Work out the finished part from the listing and answer in its coordinate system (mm). Round coordinates to 2 decimals unless told otherwise and drop trailing zeros. Write each loop counter-clockwise with the first axis right and the second up, starting at its lowest first coordinate (ties: lowest second). Pieces come first, ordered by that corner, then holes. Notation, with made-up numbers: (73.25, 60) -> (116.25, 60) arc R33 ccw to (116.25, 96) -> close; hole circle Ø5 at (1, 35.25). An arc over 180 degrees is marked (long way). One line per question, with ' | ' between items. Start each with the question number.
Autodesk Inventor part; units mm, degrees
ref_plane "YZ Plane" through (0, 0, 0) normal (1, 0, 0) x (0, 1, 0)
ref_plane "XZ Plane" through (0, 0, 0) normal (0, 1, 0) x (-1, 0, 0)
ref_plane "XY Plane" through (0, 0, 0) normal (0, 0, 1) x (1, 0, 0)
sketch "Náčrt1" plane through (0, 0, 0) normal (0, 0, 1) x (1, 0, 0)
  line L0 (0, 75) -> (0, 5)
  line L1 (145, 80) -> (5, 80)
  line L2 (5, 0) -> (145, 0)
  line L3 (150, 5) -> (150, 75)
  line L4 (21.25, 29.75) -> (21.25, 66.25)
  line L5 (21.25, 66.25) -> (36.75, 66.25)
  line L6 (36.75, 66.25) -> (36.75, 29.75)
  line L7 (36.75, 29.75) -> (21.25, 29.75)
  line L8 (41.25, 29.75) -> (41.25, 66.25)
  line L9 (56.75, 29.75) -> (41.25, 29.75)
  line L10 (56.75, 66.25) -> (56.75, 29.75)
  line L11 (41.25, 66.25) -> (56.75, 66.25)
  line L12 (140, 36) -> (68.5, 36)
  line L13 (68.5, 36) -> (68.5, 60.5)
  line L14 (68.5, 60.5) -> (140, 60.5)
  line L15 (140, 60.5) -> (140, 36)
  line L16 (74.75, 19.75) -> (74.75, 24.25)
  line L17 (79.25, 24.25) -> (79.25, 19.75)
  line L18 (74.75, 24.25) -> (79.25, 24.25)
  line L19 (79.25, 19.75) -> (74.75, 19.75)
  line L20 (90.05, 19.75) -> (85.55, 19.75)
  line L21 (85.55, 19.75) -> (85.55, 24.25)
  line L22 (85.55, 24.25) -> (90.05, 24.25)
  line L23 (90.05, 24.25) -> (90.05, 19.75)
  line L24 (96.24, 19.75) -> (96.24, 24.25)
  line L25 (96.24, 24.25) -> (100.74, 24.25)
  line L26 (100.74, 19.75) -> (96.24, 19.75)
  line L27 (100.74, 24.25) -> (100.74, 19.75)
  line L28 (107.14, 19.75) -> (107.14, 24.25)
  line L29 (107.14, 24.25) -> (111.64, 24.25)
  line L30 (111.64, 19.75) -> (107.14, 19.75)
  line L31 (111.64, 24.25) -> (111.64, 19.75)
  line L32 (117.93, 19.75) -> (117.93, 24.25)
  line L33 (117.93, 24.25) -> (122.43, 24.25)
  line L34 (122.43, 19.75) -> (117.93, 19.75)
  line L35 (122.43, 24.25) -> (122.43, 19.75)
  line L36 (128.74, 19.75) -> (128.74, 24.25)
  line L37 (128.74, 24.25) -> (133.24, 24.25)
  line L38 (133.24, 19.75) -> (128.74, 19.75)
  line L39 (133.24, 24.25) -> (133.24, 19.75)
  circle A0 centre (38.995, 70.0066) radius 1.6
  circle A1 centre (33.0004, 18.0056) radius 1.6
  circle A2 centre (37.518, 18.0056) radius 1.6
  line L40 (5, 80) -> (0, 80)
  line L41 (0, 80) -> (0, 75)
  line L42 (0, 5) -> (0, 0)
  line L43 (0, 0) -> (5, 0)
  line L44 (145, 0) -> (150, 0)
  line L45 (150, 0) -> (150, 5)
  line L46 (150, 75) -> (150, 80)
  line L47 (145, 80) -> (150, 80)
  dimension "d0" = 3.2
  dimension "d1" = 3.2
  dimension "d2" = 3.2
extrude "Vysunutí1" add sketch "Náčrt1" against normal blind 4.5
properties part number "top"
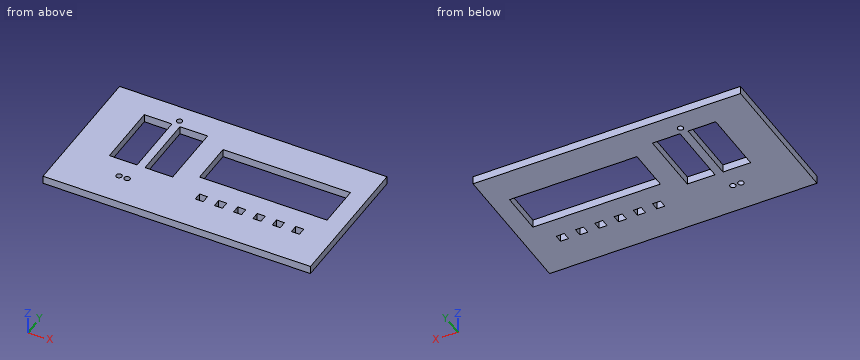
(1) A cutting plane is placed at D-D, the plane x = 92. Determine the outline of the cut face in (y, z), then the cut area to 3 significant figures.
(2) A cutting plane is placed at C-C, the plane y = 52.5. Determine the outline of the cut face in (x, z), then the cut area to 3 significant figures.
(3) Consider L1, parallel to X at y = 63, z = -1.9; L2, parallel to X at y = 51.5, z = -1.1; L3, parallel to Y at x = 87, z = -1.25. Determine where each line is inside the solid, lowest interval first.
(4) A cutting plane is placed at A-A, the plane x = 28. Determine the outline of the cut face in (y, z), then the cut area to 3 significant figures.
(5) A cutting plane is placed at B-B, the plane y = 31.5. Determine the outline of the cut face in (x, z).
Returned:
1) outline: (0, -4.5) -> (36, -4.5) -> (36, 0) -> (0, 0) -> close; (60.5, -4.5) -> (80, -4.5) -> (80, 0) -> (60.5, 0) -> close | area: 250 mm2
2) outline: (0, -4.5) -> (21.25, -4.5) -> (21.25, 0) -> (0, 0) -> close; (36.75, -4.5) -> (41.25, -4.5) -> (41.25, 0) -> (36.75, 0) -> close; (56.75, -4.5) -> (68.5, -4.5) -> (68.5, 0) -> (56.75, 0) -> close; (140, -4.5) -> (150, -4.5) -> (150, 0) -> (140, 0) -> close | area: 214 mm2
3) L1: 0 to 21.25, 36.75 to 41.25, 56.75 to 150 | L2: 0 to 21.25, 36.75 to 41.25, 56.75 to 68.5, 140 to 150 | L3: 0 to 19.75, 24.25 to 36, 60.5 to 80
4) outline: (0, -4.5) -> (29.75, -4.5) -> (29.75, 0) -> (0, 0) -> close; (66.25, -4.5) -> (80, -4.5) -> (80, 0) -> (66.25, 0) -> close | area: 196 mm2
5) outline: (0, -4.5) -> (21.25, -4.5) -> (21.25, 0) -> (0, 0) -> close; (36.75, -4.5) -> (41.25, -4.5) -> (41.25, 0) -> (36.75, 0) -> close; (56.75, -4.5) -> (150, -4.5) -> (150, 0) -> (56.75, 0) -> close
